Check sheet for the modelled part. Datum: model origin and axes. Units: mm. A direction names the side the tool comes from. Round coordinates to 2 decimals unless told otherwise and drop trailing zeros. Write each loop counter-clockwise with the first axis right and the second up, starting at its lowest first coordinate (ties: lowest second). Pieces come first, ordered by that corner, then holes. Notation, with made-up numbers: M -13.5,-1.75 L 13.5,-1.75 A20 ccw 13.5,29.25 Z; hole C -2,79 d11. An arc over 180 degrees is marked long. Put each result on its own line as item: value.
```python
from build123d import *

# Parameters (mm, degrees)
F0_R     = 11
F1_DEPTH = 5
F0_R_2   = 13.5
F2_DEPTH = 2
F3_T     = 1
F4_R     = 0.3407547834
F4_R_2   = 0.295229786
F4_R_3   = 0.330794191
F4_R_4   = 0.5
F5_DEPTH = 126.8


# Not quite as in the source:
# - a shell that OpenCascade refuses in one call is made with other operations: the cavity is built on its own and cut out


with BuildPart() as f1:
    # F0 (on Top) → F1 (new body)
    with BuildSketch(Plane.XY):
        Circle(F0_R)
    extrude(amount=F1_DEPTH)

    # F0 (on Top) → F2 (join)
    with BuildSketch(Plane.XY):
        Circle(F0_R_2)
        Circle(F0_R, mode=Mode.SUBTRACT)
    extrude(amount=F2_DEPTH)

    # F3: shell of thickness 1, made by hand


with BuildPart() as f3_core1:
    # F3_t2: copy of F1
    add(f1.part)

    # the walls: a layer under each face that stays
    f3_faces = [f3_core1.faces().sort_by_distance(p)[0] for p in [
        (-11, 0, 3.5),
        (-9, -9, 2),
        (-13.5, 0, 1),
        (0, 0, 0),
    ]]
    thicken(f3_faces, amount=-F3_T, mode=Mode.SUBTRACT)

    # F3_s3 → F3_t4 (revolve, cut)
    with BuildSketch(Plane.XZ):
        Polygon((11.01, 2.01), (10, 2), (10, 1), (11, 1), align=None)
    revolve(axis=Axis((0, 0, 2), (0, 0, 1)), mode=Mode.SUBTRACT)


with BuildPart() as f1_1:
    add(f1.part)

    # what is left inside the walls is the cavity
    f3_cavity = [f3_core1.part.solids().sort_by_distance(p)[0] for p in [
        (0, -3.333333, 1.01),
    ]]
    add(f3_cavity, mode=Mode.SUBTRACT)

    # F4 (on face) → F5 (cut, symmetric)
    with BuildSketch(Plane.XY):
        with Locations((-12.5, 0)):
            Circle(F4_R)
        with Locations((12.5, 0)):
            Circle(F4_R_2)
        with Locations((0, 12.5)):
            Circle(F4_R_3)
        with Locations((0, -12.5)):
            Circle(F4_R_4)
    extrude(amount=F5_DEPTH, both=True, mode=Mode.SUBTRACT)


solid = f1_1.part
```
1. Cross-section at D-D (y = 8.75). Enter the section's corners in (x, z).
Computed values:
outline: M -10.28,0 L 10.28,0 L 10.28,2 L 6.67,2 L 6.67,5 L 4.84,5 L 4.84,1 L -4.84,1 L -4.84,5 L -6.67,5 L -6.67,2 L -10.28,2 Z
2. Scan lines: probe 1 along Y at (x, z) = (0, 1.45); probe 2 along Y at (x, z) = (0, 0.95); probe 3 along Y at (x, z) = (0, 2.7). Record each from-to range of solid material in increasing order.
Computed values:
probe 1: y = -13.5 to -13, -12 to -10, 10 to 12.17, 12.83 to 13.5
probe 2: y = -13.5 to -13, -12 to 12.17, 12.83 to 13.5
probe 3: y = -11 to -10, 10 to 11
3. Cross-section at B-B (x = -12.5). Enter the section's corners in (y, z), then the cut area to 3 significant figures.
Computed values:
outline: M -5.1,0 L -0.34,0 L -0.34,2 L -5.1,2 Z; M 0.34,0 L 5.1,0 L 5.1,2 L 0.34,2 Z
area: 19.0 mm2
4. Cross-section at C-C (z = 3.6). Enter the section's corners in (x, y).
Computed values:
outline: C 0,0 d22; hole C 0,0 d20
5. Cross-section at A-A (x = 0). Enter the section's corners in (y, z).
Computed values:
outline: M -13.5,0 L -13,0 L -13,2 L -13.5,2 Z; M -12,0 L 12.17,0 L 12.17,2 L 11,2 L 11,5 L 10,5 L 10,1 L -10,1 L -10,5 L -11,5 L -11,2 L -12,2 Z; M 12.83,0 L 13.5,0 L 13.5,2 L 12.83,2 Z
6. Release check for a two-part mould opening along Y. For faces 3 (the cylindrical face through (0, -13, 1)), 4 (the cylindrical face through (-2.38, -10.74, 3.48)), 5 (the flat face through (2, -11, 2)), 6 (the cylindrical face through (-2.17, -9.76, 2.97)) record: +Y half, -Y half, draft (parallel to the pull), parting line (faces both ways), or undercut.
Computed values:
face 3: undercut
face 4: parting line
face 5: draft
face 6: undercut
7. Depth check by flat-ended pin: pin 1 Ø3 at (y, z) = (4.5, 2.5) entering from +X; pin 2 Ø8 at (x, y) = (1.5, -3.5) entering from +Z; pin 3 Ø1 at (y, z) = (8, 3.5) entering from -X. Enter the tip coordinate at first touch or a pass-through.
Computed values:
pin 1: stops at x = 13.14
pin 2: stops at z = 1
pin 3: stops at x = -8.05
8. Access from +Z, -Z, +X, -X, +Y, -Y to the whole of each face (thin tool, end or side, straight path). Record for faces 1 (the flat face through (0, 0, 1)), 2 (the cylindrical face through (-2.93, -13.18, 0.99)).
Computed values:
face 1: +Z
face 2: +Z, -Z
